Part print with two shaded views. Sizes in mm from the minimum x, y, z corner. A direction names the side the tool comes from. Round coordinates to 2 decimals unless told otherwise and drop trailing zeros. Write each loop counter-clockwise with the first axis right and the second up, starting at its lowest first coordinate (ties: lowest second). Pieces come first, ordered by that corner, then holes. Notation, with made-up numbers: (53, -24.5) -> (83, -24.5) arc R16 ccw to (83, -10.5) -> close; hole circle Ø4 at (5.5, 86.5). An arc over 180 degrees is marked (long way). Return JSON: item names as keys, results as strings.
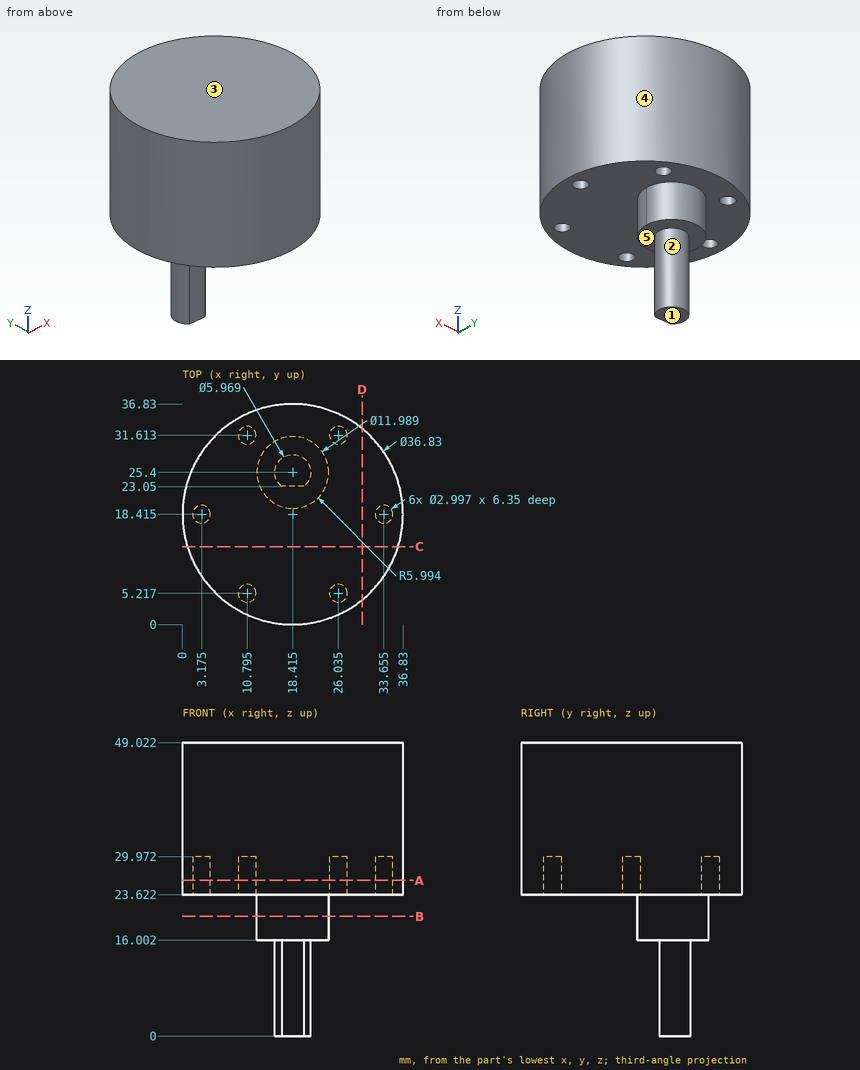
Q1. Two-plate mould, pull along Z, no slides. Class the marked faces 3, 4 and 5: +Z half, -Z half, draft (parallel to the pull), parting line (faces both ways), or undercut.
Verdict:
{"face 3": "+Z half", "face 4": "draft", "face 5": "-Z half"}
Q2. Saw through at B-B on z = 20. List the corners of the cut face in (x, y) (1 decimal), then the cut area to 3 significant figures.
Verdict:
{"outline": "circle Ø12 at (18.4, 25.4)", "area": "113 mm²"}
Q3. 3-axis set-ups, long thin cutter, end or side, ignore diameter. For the marked faces 1 and 2: which of +Z, -Z, +X, -X, +Y, -Y reach the whole face in a straight line?
Verdict:
{"face 1": "-Z, +X, -X, +Y, -Y", "face 2": "-Z"}
Q4. Pin check, flat tips, straight feed: pin 1 Ø5 at (x, z) = (31, 35) entering from -Y; pin 2 Ø2.5 at (x, y) = (34, 18.5) entering from -Z; pin 3 Ø8 at (y, z) = (23, 6.5) entering from +X. Stop position of each tip, or through.
Verdict:
{"pin 1": "stops at y = 3.01", "pin 2": "stops at z = 23.62", "pin 3": "stops at x = 21.4"}
Q5. Saw through at D-D on x = 30. List the corners of the cut face in (y, z).
Verdict:
{"outline": "(4.1, 23.62) -> (32.73, 23.62) -> (32.73, 49.02) -> (4.1, 49.02) -> close"}
Q6. Saw through at A-A on z = 26. List the corners of the cut face in (x, y) (1 decimal).
Verdict:
{"outline": "circle Ø36.8 at (18.4, 18.4); hole circle Ø3 at (3.2, 18.4); hole circle Ø3 at (10.8, 5.2); hole circle Ø3 at (10.8, 31.6); hole circle Ø3 at (26, 5.2); hole circle Ø3 at (26, 31.6); hole circle Ø3 at (33.7, 18.4)"}
Q7. Saw through at C-C on y = 13. List the corners of the cut face in (x, z) (1 decimal), then the cut area to 3 significant figures.
Verdict:
{"outline": "(0.8, 23.6) -> (36, 23.6) -> (36, 49) -> (0.8, 49) -> close", "area": "894 mm²"}
Q8. Wall check: L1, parallel to X at y = 19, z = 44.5; L2, parallel to Z at x = 24, y = 7; L3, parallel to Z at x = 34, y = 18. Give the ranges that are in metal, low to high.
Verdict:
{"L1": "x = 0.01 to 36.82", "L2": "z = 23.62 to 49.02", "L3": "z = 29.97 to 49.02"}
